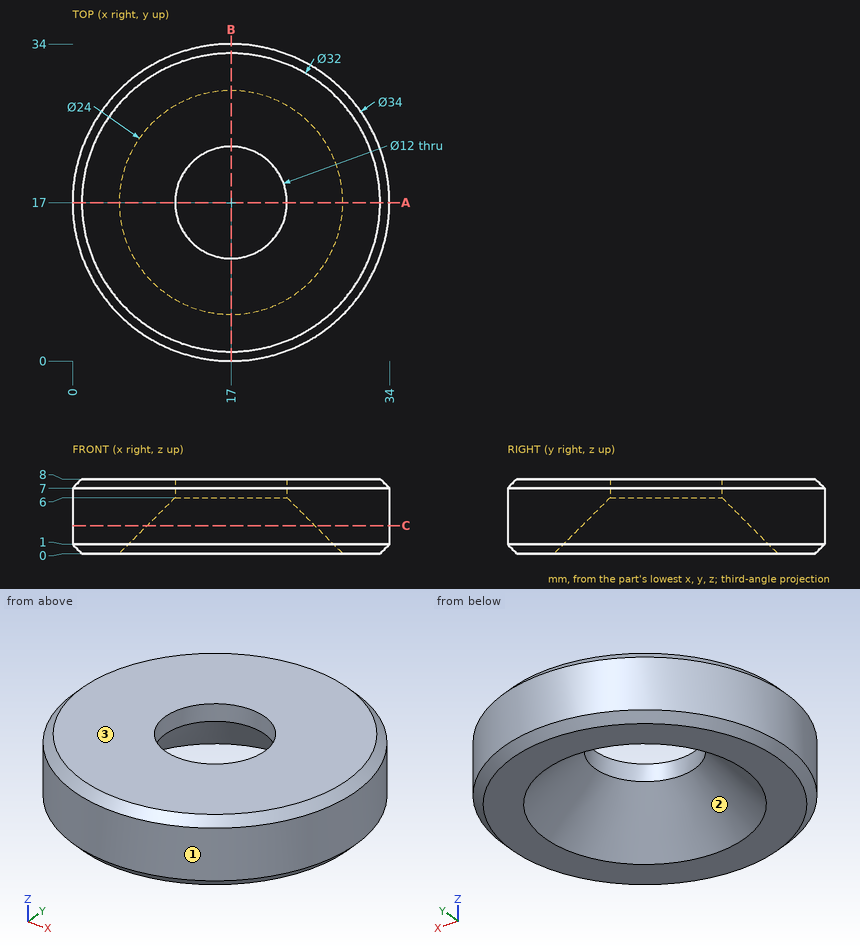
Print and shaded views of the part. All mm, measured from the part's lowest x, y and z. Give positions to 0.01 mm unless a question says otherwise; leave off trailing zeros. Order: outer loops, then holes, each group sorted by start corner. A loop starts at its lowest first (then second) coordinate and runs counter-clockwise, first axis right, second up. Notation, with made-up numbers: (7, -37.75) - (49, -37.75) arc R27 ccw to (49, -12.75) - close; hole circle Ø10 at (59, 54.5). An arc over 180 degrees is marked (long way). One line per item, written item: value.
Item 1: Pin check, flat tips, straight feed: pin 1 Ø1.5 at (y, z) = (11.5, 3) entering from +X; pin 2 Ø3 at (x, z) = (5.5, 4.5) entering from +Y; pin 3 Ø1.5 at (x, z) = (9, 5) entering from -Y. Stop position of each tip, or through.
Response values:
pin 1: x = 33.32
pin 2: y = 30.75
pin 3: y = 1.62
Item 2: Slice it at A-A (y = 17). List the corners of the cut face in (x, z).
Response values:
outline: (0, 1) - (1, 0) - (5, 0) - (11, 6) - (11, 8) - (1, 8) - (0, 7) - close; (23, 6) - (29, 0) - (33, 0) - (34, 1) - (34, 7) - (33, 8) - (23, 8) - close
Item 3: Two-plate mould, pull along X, no slides. Class the marked faces 1, 2 and 3: released by +X, released by -X, zero draft, split by the parting line, or undercut.
Response values:
face 1: split by the parting line
face 2: undercut
face 3: zero draft
Item 4: Slice it at C-C (z = 3). List the corners of the cut face in (x, y), then the cut area to 3 significant figures.
Response values:
outline: circle Ø34 at (17, 17); hole circle Ø18 at (17, 17)
area: 653 mm2
Item 5: Wall check: line 1 (Y direction, x = 17, z = 6.85); line 2 (X direction, y = 25, z = 0.5); line 3 (Y direction, x = 19.5, z = 5). Give the ranges that are in metal, low to high.
Response values:
line 1: 0 to 11, 23 to 34
line 2: 2.57 to 8.74, 25.26 to 31.43
line 3: 0.18 to 10.46, 23.54 to 33.82
